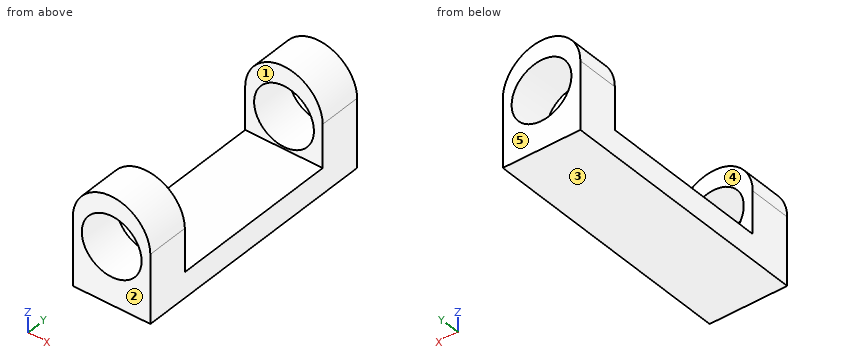
```python
from build123d import *

# Parameters (mm, degrees)
F1_DEPTH = 30
F2_R     = 3.5
F3_DEPTH = 30.001
F4_W     = 20
F4_H     = 10.027466
F5_DEPTH = 9.075462


with BuildPart() as f1:
    # F0 (on Front) → F1 (new body)
    with BuildSketch(Plane.XZ):
        with BuildLine():
            Line((0, 7.925374), (0, 0))
            Line((0, 0), (9.074462, 0))
            Line((9.074462, 0), (9.074462, 8))
            ThreePointArc((9.074462, 8), (4.500224, 12.462759), (0, 7.925374))
        make_face()
    extrude(amount=F1_DEPTH)

    # F2 (on Front) → F3 (cut, through all)
    with BuildSketch(Plane.XZ):
        with Locations((4.548298, 6.713609)):
            Circle(F2_R)
    extrude(amount=F3_DEPTH, mode=Mode.SUBTRACT)

    # F4 (on Right) → F5 (cut, through all)
    with BuildSketch(Plane.YZ):
        with Locations((-15, 7.985694)):
            Rectangle(F4_W, F4_H)
    extrude(amount=F5_DEPTH, mode=Mode.SUBTRACT)


solid = f1.part
```
Work out the finished part from the listing and answer in its coordinate system (mm). Face numbers are marked on the shaded views. A direction names the side the tool comes from. Coordinates: 2 decimals unless noted, no trailing zeros. Order: outer loops, then holes, each group sorted by start corner. A loop starts at its lowest first (then second) coordinate and runs counter-clockwise, first axis right, second up. Notation, with made-up numbers: (76.5, 77.5) - (88.5, 77.5) arc R27 cw to (88.5, 94.5) - close; hole circle Ø7 at (8.5, -8.5). An arc over 180 degrees is marked (long way). Answer as a JSON object with one key per item and string values.
1. Find section B-B on z = 11. Determine the outline of the cut face in (x, y).
Output values:
{"outline": "(1.2, -30) - (7.87, -30) - (7.87, -25) - (1.2, -25) - close; (1.2, -5) - (7.87, -5) - (7.87, 0) - (1.2, 0) - close"}
2. Consider line 1 (Y direction, x = 7, z = 11.5); line 2 (Z direction, x = 5.25, y = -3.75); line 3 (X direction, y = -26.5, z = 5.5). Determine where each line is inside the solid, lowest interval first.
Output values:
{"line 1": "y = -30 to -25, -5 to 0", "line 2": "z = 0 to 3.28, 10.14 to 12.41", "line 3": "x = 0 to 1.27, 7.83 to 9.07"}
3. Find section A-A on z = 3.5. Determine the outline of the cut face in (x, y).
Output values:
{"outline": "(0, -30) - (3.16, -30) - (3.16, -25) - (0, -25) - close; (0, -5) - (3.16, -5) - (3.16, 0) - (0, 0) - close; (5.93, -30) - (9.07, -30) - (9.07, -25) - (5.93, -25) - close; (5.93, -5) - (9.07, -5) - (9.07, 0) - (5.93, 0) - close"}
4. This flat-tipped pin is pushed along its axis until it touches: P1, Ø2, axis at x = 1.5, y = -17, coming from the +Z side. Where does it stop, or does it pass through?
Output values:
{"P1": "stops at z = 2.97"}
5. A tool of negligible diameter and unlimited length cuts with its end or side. For the marked faces 4 and 5, from which of +Z, -Z, +X, -X, +Y, -Y can it reach the whole face along a straight path? Write none if from no direction.
Output values:
{"face 4": "+Z, +X, -X", "face 5": "+Z, -Z, +X, -X, +Y"}
6. Find section C-C on x = 2.75. Determine the outline of the cut face in (y, z).
Output values:
{"outline": "(-30, 0) - (0, 0) - (0, 3.71) - (-5, 3.71) - (-5, 2.97) - (-25, 2.97) - (-25, 3.71) - (-30, 3.71) - close; (-30, 9.72) - (-25, 9.72) - (-25, 12.1) - (-30, 12.1) - close; (-5, 9.72) - (0, 9.72) - (0, 12.1) - (-5, 12.1) - close"}
7. The mould has two halves that part along Y. Classify the marked faces 1, 2 and 3: +Y half, -Y half, draft (parallel to the pull), parting line (faces both ways), or undercut.
Output values:
{"face 1": "undercut", "face 2": "-Y half", "face 3": "draft"}
